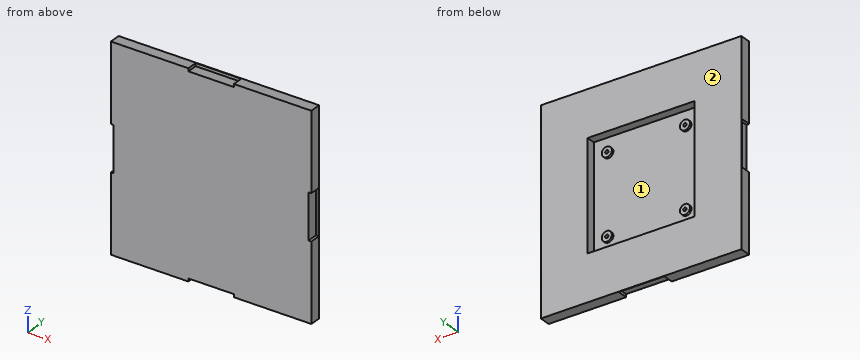
```python
from build123d import *

# Parameters (mm, degrees)
SKETCH1_W           = 180
SKETCH1_H           = 180
SKETCH1_W_2         = 96.073021888
SKETCH1_H_2         = 97.47003078
BOSS_EXTRUDE1_DEPTH = 10
SKETCH1_3_W         = 96.073021888
SKETCH1_3_H         = 97.47003078
SKETCH1_3_R         = 4.5
BOSS_EXTRUDE2_DEPTH = 2
SKETCH1_5_R         = 1.5
BOSS_EXTRUDE3_DEPTH = 4
CUT_EXTRUDE1_START  = 4
SKETCH1_6_R         = 1.5
CUT_EXTRUDE1_DEPTH  = 2.5
SKETCH4_W           = 40
SKETCH4_H           = 9
CUT_EXTRUDE3_DEPTH  = 2.6
CIRPATTERN2_COUNT   = 4


with BuildPart() as part:
    # Sketch1 → Boss-Extrude1 (new body)
    with BuildSketch(Plane(origin=(0, 0, 0), x_dir=(1, 0, 0), z_dir=(0, 1, 0))):
        Rectangle(SKETCH1_W, SKETCH1_H)
        Rectangle(SKETCH1_W_2, SKETCH1_H_2, mode=Mode.SUBTRACT)
    extrude(amount=BOSS_EXTRUDE1_DEPTH)

    # Sketch1<3> → Boss-Extrude2 (add)
    with BuildSketch(Plane(origin=(0, 0, 0), x_dir=(1, 0, 0), z_dir=(0, 1, 0))):
        Rectangle(SKETCH1_3_W, SKETCH1_3_H)
        with Locations(Location((34.990916942, 35.687000466, 0), (0, 0, 270))):
            Circle(SKETCH1_3_R, mode=Mode.SUBTRACT)
        with Locations(Location((34.990916942, -35.558880992, 0), (0, 0, 270))):
            Circle(SKETCH1_3_R, mode=Mode.SUBTRACT)
        with Locations(Location((-35.115505573, -35.558880992, 0), (0, 0, 270))):
            Circle(SKETCH1_3_R, mode=Mode.SUBTRACT)
        with Locations(Location((-35.115505573, 35.687000466, 0), (0, 0, 270))):
            Circle(SKETCH1_3_R, mode=Mode.SUBTRACT)
    extrude(amount=BOSS_EXTRUDE2_DEPTH)

    # Sketch1<5> → Boss-Extrude3 (add)
    # profile 1 of 12: a face of its own
    with BuildSketch(Plane(origin=(0, 0, 0), x_dir=(1, 0, 0), z_dir=(0, 1, 0))):
        with BuildLine():
            Line((-38.036510944, -38.73501539), (-38.036510944, -32.135764339))
            ThreePointArc((-38.036510944, -32.135764339), (-38.417826814, -38.615787014), (-31.927689662, -38.73501539))
            Line((-31.927689662, -38.73501539), (-38.036510944, -38.73501539))
        make_face()
    # profile 2 of 12: a face of its own
    with BuildSketch(Plane(origin=(0, 0, 0), x_dir=(1, 0, 0), z_dir=(0, 1, 0))):
        with BuildLine():
            ThreePointArc((-30.615505573, -35.558880992), (-33.230634778, -31.472652647), (-38.036510944, -32.135764339))
            Line((-38.036510944, -32.135764339), (-38.036510944, -38.73501539))
            Line((-38.036510944, -38.73501539), (-31.927689662, -38.73501539))
            ThreePointArc((-31.927689662, -38.73501539), (-30.95646893, -37.277140053), (-30.615505573, -35.558880992))
        make_face()
        with Locations((-35.115505573, -35.558880992)):
            Circle(SKETCH1_5_R, mode=Mode.SUBTRACT)
    # profile 3 of 12: a face of its own
    with BuildSketch(Plane(origin=(0, 0, 0), x_dir=(1, 0, 0), z_dir=(0, 1, 0))):
        with Locations((-35.115505573, -35.558880992)):
            Circle(SKETCH1_5_R)
    # profile 4 of 12: a face of its own
    with BuildSketch(Plane(origin=(0, 0, 0), x_dir=(1, 0, 0), z_dir=(0, 1, 0))):
        with BuildLine():
            Line((38.036510944, -38.73501539), (38.036510944, -32.246124259))
            ThreePointArc((38.036510944, -32.246124259), (31.745692174, -32.441427511), (31.80310103, -38.73501539))
            Line((31.80310103, -38.73501539), (38.036510944, -38.73501539))
        make_face()
        with Locations((34.990916942, -35.558880992)):
            Circle(SKETCH1_5_R, mode=Mode.SUBTRACT)
    # profile 5 of 12: a face of its own
    with BuildSketch(Plane(origin=(0, 0, 0), x_dir=(1, 0, 0), z_dir=(0, 1, 0))):
        with Locations((34.990916942, -35.558880992)):
            Circle(SKETCH1_5_R)
    # profile 6 of 12: a face of its own
    with BuildSketch(Plane(origin=(0, 0, 0), x_dir=(1, 0, 0), z_dir=(0, 1, 0))):
        with BuildLine():
            ThreePointArc((39.490916942, -35.558880992), (39.111303636, -33.74989965), (38.036510944, -32.246124259))
            Line((38.036510944, -32.246124259), (38.036510944, -38.73501539))
            Line((38.036510944, -38.73501539), (31.80310103, -38.73501539))
            ThreePointArc((31.80310103, -38.73501539), (36.709176002, -39.717917636), (39.490916942, -35.558880992))
        make_face()
    # profile 7 of 12: a face of its own
    with BuildSketch(Plane(origin=(0, 0, 0), x_dir=(1, 0, 0), z_dir=(0, 1, 0))):
        with BuildLine():
            Line((-31.804976156, 38.73501539), (-38.036510944, 38.73501539))
            Line((-38.036510944, 38.73501539), (-38.036510944, 32.263883812))
            ThreePointArc((-38.036510944, 32.263883812), (-33.230634778, 31.600772121), (-30.615505573, 35.687000466))
            ThreePointArc((-30.615505573, 35.687000466), (-30.923406912, 37.322943255), (-31.804976156, 38.73501539))
        make_face()
        with Locations((-35.115505573, 35.687000466)):
            Circle(SKETCH1_5_R, mode=Mode.SUBTRACT)
    # profile 8 of 12: a face of its own
    with BuildSketch(Plane(origin=(0, 0, 0), x_dir=(1, 0, 0), z_dir=(0, 1, 0))):
        with Locations((-35.115505573, 35.687000466)):
            Circle(SKETCH1_5_R)
    # profile 9 of 12: a face of its own
    with BuildSketch(Plane(origin=(0, 0, 0), x_dir=(1, 0, 0), z_dir=(0, 1, 0))):
        with BuildLine():
            Line((-38.036510944, 32.263883812), (-38.036510944, 38.73501539))
            Line((-38.036510944, 38.73501539), (-31.804976156, 38.73501539))
            ThreePointArc((-31.804976156, 38.73501539), (-38.356927826, 38.808407485), (-38.036510944, 32.263883812))
        make_face()
    # profile 10 of 12: a face of its own
    with BuildSketch(Plane(origin=(0, 0, 0), x_dir=(1, 0, 0), z_dir=(0, 1, 0))):
        with BuildLine():
            Line((38.036510944, 38.73501539), (31.680387525, 38.73501539))
            ThreePointArc((31.680387525, 38.73501539), (31.807773572, 32.50618323), (38.036510944, 32.374243733))
            Line((38.036510944, 32.374243733), (38.036510944, 38.73501539))
        make_face()
        with Locations((34.990916942, 35.687000466)):
            Circle(SKETCH1_5_R, mode=Mode.SUBTRACT)
    # profile 11 of 12: a face of its own
    with BuildSketch(Plane(origin=(0, 0, 0), x_dir=(1, 0, 0), z_dir=(0, 1, 0))):
        with Locations((34.990916942, 35.687000466)):
            Circle(SKETCH1_5_R)
    # profile 12 of 12: a face of its own
    with BuildSketch(Plane(origin=(0, 0, 0), x_dir=(1, 0, 0), z_dir=(0, 1, 0))):
        with BuildLine():
            ThreePointArc((39.490916942, 35.687000466), (36.626859732, 39.879099127), (31.680387525, 38.73501539))
            Line((31.680387525, 38.73501539), (38.036510944, 38.73501539))
            Line((38.036510944, 38.73501539), (38.036510944, 32.374243733))
            ThreePointArc((38.036510944, 32.374243733), (39.111303636, 33.878019124), (39.490916942, 35.687000466))
        make_face()
    extrude(amount=BOSS_EXTRUDE3_DEPTH)

    # Sketch1<6> → Cut-Extrude1 (cut)
    with BuildSketch(Plane(origin=(0, 0, 0), x_dir=(1, 0, 0), z_dir=(0, 1, 0)).offset(CUT_EXTRUDE1_START)):
        with Locations(Location((-35.115505573, 35.687000466, 0), (0, 0, 270))):
            Circle(SKETCH1_6_R)
        with Locations(Location((34.990916942, 35.687000466, 0), (0, 0, 270))):
            Circle(SKETCH1_6_R)
        with Locations(Location((34.990916942, -35.558880992, 0), (0, 0, 270))):
            Circle(SKETCH1_6_R)
        with Locations(Location((-35.115505573, -35.558880992, 0), (0, 0, 270))):
            Circle(SKETCH1_6_R)
    extrude(amount=-CUT_EXTRUDE1_DEPTH, mode=Mode.SUBTRACT)

    # Sketch4 → Cut-Extrude3 (cut)
    with BuildSketch(Plane(origin=(0, 0, -90), x_dir=(-1, 0, 0), z_dir=(0, 0, -1))):
        Polygon((-20, 0), (-20, 9), (20, 9), (20, 0), (20.4, 0), (20.4, 9.4), (-20.4, 9.4), (-20.4, 0), align=None)
        with Locations((0, 4.5)):
            Rectangle(SKETCH4_W, SKETCH4_H)
    cut_extrude3 = extrude(amount=-CUT_EXTRUDE3_DEPTH, mode=Mode.SUBTRACT)

    # CirPattern2: Cut-Extrude3 ×4 about axis
    cirpattern2_axis = Axis((0.001740107, 0, 0.001789421), (0, 1, 0))
    for i in range(1, CIRPATTERN2_COUNT):
        add(cut_extrude3.rotate(cirpattern2_axis, i * 360 / CIRPATTERN2_COUNT), mode=Mode.SUBTRACT)


solid = part.part
```
Here's how the part is built. I have some questions about the finished solid (model axes, mm). Face numbers are marked on the shaded views. Round coordinates to 2 decimals unless told otherwise and drop trailing zeros. Order: outer loops, then holes, each group sorted by start corner. A loop starts at its lowest first (then second) coordinate and runs counter-clockwise, first axis right, second up. Notation, with made-up numbers: (9, 15.25) -> (23, 15.25) arc R22 cw to (23, 48.25) -> close; hole circle Ø4 at (60, 41.5). An arc over 180 degrees is marked (long way). Use a Markdown table: item, result. Add a question column.
(1) Suppose I cut it at B-B, the plane x = -27. Please give me the cut outline in (y, z).
(2) Suppose I cut it at C-C, the plane z = 8. Please give me the cut outline in (x, y).
(3) I need wall thicknesses on line 1 along Z through (x, y) = (-9, 9.25); line 2 along X through (y, z) = (5.25, 20); line 3 along X through (y, z) = (7.75, -48). Which ranges of each line are inside material? Lowest first, please.
(4) Suppose I cut it at A-A, the plane z = 26. Please give me the cut outline in (x, y), and give its area (3 significant figures).
(5) Suppose I cut it at D-D, the plane x = -4. Please give me the cut outline in (y, z), and give its area (3 significant figures).
(6) For pin 1 Ø1 at (x, z) = (33, -8) entering from -Y; pin 2 Ø12 at (x, z) = (41.5, 9) entering from +Y; pin 3 Ø2.5 at (x, y) = (-15, 5) entering from +Z; pin 4 Ø4.5 at (y, z) = (2.5, -7.5) entering from +X, each with a flat end and sliding along its axis, tell me the tip position at first contact or that it passes through.
(7) If we mould it in two halves opening along Z, with no side actions, what happens to the marked faces 1 and 2? For each: released by +Z, released by -Z, zero draft, split by the parting line, or undercut.
Verdict:
| question | item | result |
|---|---|---|
| 1 | outline | (0, -90) -> (10, -90) -> (10, -48.74) -> (2, -48.74) -> (2, 48.74) -> (10, 48.74) -> (10, 90) -> (0, 90) -> close |
| 2 | outline | (-90, 9.4) -> (-87.4, 9.4) -> (-87.4, 0) -> (87.4, 0) -> (87.4, 9.4) -> (90, 9.4) -> (90, 10) -> (48.04, 10) -> (48.04, 2) -> (-48.04, 2) -> (-48.04, 10) -> (-90, 10) -> close |
| 3 | line 1 | -87.4 to -48.74, 48.74 to 87.4 |
| 3 | line 2 | -87.4 to -48.04, 48.04 to 87.4 |
| 3 | line 3 | -90 to -48.04, 48.04 to 90 |
| 4 | outline | (-90, 0) -> (90, 0) -> (90, 10) -> (48.04, 10) -> (48.04, 2) -> (-48.04, 2) -> (-48.04, 10) -> (-90, 10) -> close |
| 4 | area | 1,030 mm2 |
| 5 | outline | (0, -87.4) -> (9.4, -87.4) -> (9.4, -90) -> (10, -90) -> (10, -48.74) -> (2, -48.74) -> (2, 48.74) -> (10, 48.74) -> (10, 90) -> (9.4, 90) -> (9.4, 87.4) -> (0, 87.4) -> close |
| 5 | area | 971 mm2 |
| 6 | pin 1 | y = 0 |
| 6 | pin 2 | y = 2 |
| 6 | pin 3 | z = 87.4 |
| 6 | pin 4 | x = 87.4 |
| 7 | face 1 | undercut |
| 7 | face 2 | zero draft |
